```python
from build123d import *

# Parameters (mm, degrees)
SKETCH2_W           = 50.8
SKETCH2_H           = 25.4
BOSS_EXTRUDE1_DEPTH = 3.175
SKETCH4_W           = 38.1
SKETCH4_H           = 50.8
BOSS_EXTRUDE2_DEPTH = 3.175
SKETCH5_R           = 1.1
CUT_EXTRUDE1_DEPTH  = 3.175
SKETCH6_R           = 3.175
CUT_EXTRUDE2_DEPTH  = 3.175
BOSS_EXTRUDE3_DEPTH = 1.5875
FILLET3_R           = 1.5


with BuildPart() as part:
    # Sketch2 → Boss-Extrude1 (new body)
    with BuildSketch(Plane(origin=(0, 0, 0), x_dir=(0, 0, -1), z_dir=(1, 0, 0))):
        Rectangle(SKETCH2_W, SKETCH2_H)
    extrude(amount=BOSS_EXTRUDE1_DEPTH)

    # Sketch4 → Boss-Extrude2 (add)
    with BuildSketch(Plane(origin=(0, 12.7, 0), x_dir=(1, 0, 0), z_dir=(0, 1, 0))):
        with Locations((19.05, 0)):
            Rectangle(SKETCH4_W, SKETCH4_H)
    extrude(amount=-BOSS_EXTRUDE2_DEPTH)

    # Sketch5 → Cut-Extrude1 (cut)
    with BuildSketch(Plane(origin=(0, 12.7, 0), x_dir=(1, 0, 0), z_dir=(0, 1, 0))):
        with Locations(Location((8.05, 18.5, 0), (0, 0, 270))):
            Circle(SKETCH5_R)
        with Locations(Location((34.05, 18.5, 0), (0, 0, 270))):
            Circle(SKETCH5_R)
        with Locations(Location((34.05, -18.5, 0), (0, 0, 270))):
            Circle(SKETCH5_R)
        with Locations(Location((8.05, -18.5, 0), (0, 0, 270))):
            Circle(SKETCH5_R)
    extrude(amount=-CUT_EXTRUDE1_DEPTH, mode=Mode.SUBTRACT)

    # Sketch6 → Cut-Extrude2 (cut)
    with BuildSketch(Plane.ZY):
        with Locations((-12.7, 0)):
            Circle(SKETCH6_R)
        with Locations((12.7, 0)):
            Circle(SKETCH6_R)
    extrude(amount=-CUT_EXTRUDE2_DEPTH, mode=Mode.SUBTRACT)

    # Sketch7 → Boss-Extrude3 (add, symmetric)
    with BuildSketch(Plane.XY):
        Polygon((3.175, -12.7), (25.4, 9.525), (3.175, 9.525), align=None)
    extrude(amount=BOSS_EXTRUDE3_DEPTH, both=True)

    # Fillet3
    # the kernel refuses this fillet: 1.5 mm, written as the material it adds along each edge
    with BuildSketch(Plane(origin=(4.675, 8.025, 3.0875), x_dir=(-1, 0, 0), z_dir=(0, 1, 0))) as fillet3_piece_1_section:
        Polygon((0, 0), (FILLET3_R, 0), (FILLET3_R, -FILLET3_R), (0, -FILLET3_R), align=None)
    fillet3_piece_1 = extrude(amount=FILLET3_R, mode=Mode.PRIVATE)
    fillet3_piece_1 = fillet3_piece_1 - Plane(origin=(4.675, 8.025, 3.0875), x_dir=(0.7071067811865475, 0, 0.7071067811865475), z_dir=(0, 1, 0)) * Sphere(FILLET3_R, mode=Mode.PRIVATE)
    add(fillet3_piece_1)
    with BuildSketch(Plane(origin=(4.675, 8.025, -3.0875), x_dir=(0, 0, 1), z_dir=(0, 1, 0))) as fillet3_piece_2_section:
        Polygon((0, 0), (FILLET3_R, 0), (FILLET3_R, -FILLET3_R), (0, -FILLET3_R), align=None)
    fillet3_piece_2 = extrude(amount=FILLET3_R, mode=Mode.PRIVATE)
    fillet3_piece_2 = fillet3_piece_2 - Plane(origin=(4.675, 8.025, -3.0875), x_dir=(0.7071067811865475, 0, -0.7071067811865475), z_dir=(0, 1, 0)) * Sphere(FILLET3_R, mode=Mode.PRIVATE)
    add(fillet3_piece_2)
    with BuildSketch(Plane(origin=(3.175, 9.525, 25.4), x_dir=(0, -1, 0), z_dir=(0, 0, -1)), Plane(origin=(3.175, 9.525, -3.0875), x_dir=(0, -1, 0), z_dir=(0, 0, -1))) as fillet3_piece_3:
        with BuildLine():
            CenterArc((FILLET3_R, -FILLET3_R), FILLET3_R, 90, 90)
            Line((0, -FILLET3_R), (0, 0))
            Line((0, 0), (FILLET3_R, 0))
        make_face()
    extrude(amount=22.3125)
    with BuildSketch(Plane(origin=(29.15, 9.525, -1.5875), x_dir=(0, 0, -1), z_dir=(-1, 0, 0))) as fillet3_piece_4_section:
        with BuildLine():
            CenterArc((FILLET3_R, FILLET3_R), FILLET3_R, 180, 90)
            Line((0, FILLET3_R), (0, 0))
            Line((0, 0), (FILLET3_R, 0))
        make_face()
    fillet3_piece_4 = extrude(amount=24.475, mode=Mode.PRIVATE)
    fillet3_piece_4 = split(fillet3_piece_4, bisect_by=Plane(origin=(19.967902823, 4.092902823, -1.930123153), z_dir=(-0.707106781186549, 0.707106781186546, 0)), keep=Keep.TOP, mode=Mode.PRIVATE)
    add(fillet3_piece_4)
    with BuildSketch(Plane(origin=(25.4, 9.525, -1.5875), x_dir=(-0.7071067811865489, -0.7071067811865461, 0), z_dir=(0, 0, 1))) as fillet3_piece_5:
        with BuildLine():
            CenterArc((FILLET3_R * 0.414213562373, FILLET3_R), FILLET3_R, 225, 45)
            Line((-FILLET3_R * 0.292893218813, FILLET3_R * 0.292893218813), (0, 0))
            Line((0, 0), (FILLET3_R * 0.414213562373, 0))
        make_face()
    extrude(amount=3.175)
    with BuildSketch(Plane(origin=(3.175, 8.025, -1.5875), x_dir=(0, 0, -1), z_dir=(0, -1, 0))) as fillet3_piece_6_section:
        with BuildLine():
            CenterArc((FILLET3_R, FILLET3_R), FILLET3_R, 180, 90)
            Line((0, FILLET3_R), (0, 0))
            Line((0, 0), (FILLET3_R, 0))
        make_face()
    fillet3_piece_6 = extrude(amount=20.725, mode=Mode.PRIVATE)
    fillet3_piece_6 = split(fillet3_piece_6, bisect_by=Plane(origin=(8.60741784, -7.26758216, -1.930100054), z_dir=(-0.707106781186549, 0.707106781186546, 0)), keep=Keep.TOP, mode=Mode.PRIVATE)
    add(fillet3_piece_6)
    with BuildSketch(Plane(origin=(29.15, 9.525, 1.5875), x_dir=(0, 0, 1), z_dir=(-1, 0, 0))) as fillet3_piece_7_section:
        with BuildLine():
            CenterArc((FILLET3_R, -FILLET3_R), FILLET3_R, 90, 90)
            Line((0, -FILLET3_R), (0, 0))
            Line((0, 0), (FILLET3_R, 0))
        make_face()
    fillet3_piece_7 = extrude(amount=24.475, mode=Mode.PRIVATE)
    fillet3_piece_7 = split(fillet3_piece_7, bisect_by=Plane(origin=(19.967902823, 4.092902823, 1.930123153), z_dir=(-0.707106781186549, 0.707106781186546, 0)), keep=Keep.TOP, mode=Mode.PRIVATE)
    add(fillet3_piece_7)
    with BuildSketch(Plane(origin=(3.175, 8.025, 1.5875), x_dir=(0, 0, 1), z_dir=(0, -1, 0))) as fillet3_piece_8_section:
        with BuildLine():
            CenterArc((FILLET3_R, -FILLET3_R), FILLET3_R, 90, 90)
            Line((0, -FILLET3_R), (0, 0))
            Line((0, 0), (FILLET3_R, 0))
        make_face()
    fillet3_piece_8 = extrude(amount=20.725, mode=Mode.PRIVATE)
    fillet3_piece_8 = split(fillet3_piece_8, bisect_by=Plane(origin=(8.60741784, -7.26758216, 1.930100054), z_dir=(-0.707106781186549, 0.707106781186546, 0)), keep=Keep.TOP, mode=Mode.PRIVATE)
    add(fillet3_piece_8)
    with BuildSketch(Plane(origin=(25.4, 9.525, -3.140800859), x_dir=(-0.7071067811865446, -0.7071067811865503, 0), z_dir=(0, 0, 1))) as fillet3_piece_9a_section:
        with BuildLine():
            CenterArc((FILLET3_R * 0.414213562373, FILLET3_R), FILLET3_R, 225, 45)
            Line((-FILLET3_R * 0.292893218813, FILLET3_R * 0.292893218813), (0, 0))
            Line((0, 0), (FILLET3_R * 0.414213562373, 0))
        make_face()
    fillet3_piece_9a = extrude(amount=4.728300859, mode=Mode.PRIVATE)
    fillet3_piece_9a = split(fillet3_piece_9a, bisect_by=Plane(origin=(25.438403899, 9.432284787, -1.5875), z_dir=(0, 0, -1)), keep=Keep.TOP, mode=Mode.PRIVATE)
    with BuildSketch(Plane(origin=(29.15, 9.525, -1.5875), x_dir=(0, 0, -1), z_dir=(-1, 0, 0))) as fillet3_piece_9b_section:
        with BuildLine():
            CenterArc((FILLET3_R, FILLET3_R), FILLET3_R, 180, 90)
            Line((0, FILLET3_R), (0, 0))
            Line((0, 0), (FILLET3_R, 0))
        make_face()
    fillet3_piece_9b = extrude(amount=24.475, mode=Mode.PRIVATE)
    fillet3_piece_9b = split(fillet3_piece_9b, bisect_by=Plane(origin=(26.063627713, 10.188627713, -1.91198662), z_dir=(0.707106781186549, -0.707106781186546, 0)), keep=Keep.TOP, mode=Mode.PRIVATE)
    fillet3_piece_9 = fillet3_piece_9a & fillet3_piece_9b
    add(fillet3_piece_9)
    with BuildSketch(Plane(origin=(25.4, 9.525, -1.5875), x_dir=(-0.7071067811865489, -0.7071067811865461, 0), z_dir=(0, 0, 1))) as fillet3_piece_10a_section:
        with BuildLine():
            CenterArc((FILLET3_R * 0.414213562373, FILLET3_R), FILLET3_R, 225, 45)
            Line((-FILLET3_R * 0.292893218813, FILLET3_R * 0.292893218813), (0, 0))
            Line((0, 0), (FILLET3_R * 0.414213562373, 0))
        make_face()
    fillet3_piece_10a = extrude(amount=4.728300859, mode=Mode.PRIVATE)
    fillet3_piece_10a = split(fillet3_piece_10a, bisect_by=Plane(origin=(25.438403899, 9.432284787, 1.5875), z_dir=(0, 0, 1)), keep=Keep.TOP, mode=Mode.PRIVATE)
    with BuildSketch(Plane(origin=(29.15, 9.525, 1.5875), x_dir=(0, 0, 1), z_dir=(-1, 0, 0))) as fillet3_piece_10b_section:
        with BuildLine():
            CenterArc((FILLET3_R, -FILLET3_R), FILLET3_R, 90, 90)
            Line((0, -FILLET3_R), (0, 0))
            Line((0, 0), (FILLET3_R, 0))
        make_face()
    fillet3_piece_10b = extrude(amount=24.475, mode=Mode.PRIVATE)
    fillet3_piece_10b = split(fillet3_piece_10b, bisect_by=Plane(origin=(26.063627713, 10.188627713, 1.91198662), z_dir=(0.707106781186549, -0.707106781186546, 0)), keep=Keep.TOP, mode=Mode.PRIVATE)
    fillet3_piece_10 = fillet3_piece_10a & fillet3_piece_10b
    add(fillet3_piece_10)
    # the kernel refuses this fillet: 1.5 mm, written as the material it takes off along each edge
    with BuildSketch(Plane(origin=(38.1, 16.45, 25.4), x_dir=(0, 0, -1), z_dir=(0, -1, 0)), Plane(origin=(-3.75, -12.7, -25.4), x_dir=(0, 0, 1), z_dir=(1, 0, 0))) as fillet3_2_piece_1:
        with BuildLine():
            CenterArc((FILLET3_R, -FILLET3_R), FILLET3_R, 90, 90)
            Line((0, -FILLET3_R), (0, 0))
            Line((0, 0), (FILLET3_R, 0))
        make_face()
    extrude(amount=10.675, mode=Mode.SUBTRACT)
    with BuildSketch(Plane(origin=(38.1, 16.45, -25.4), x_dir=(0, 0, 1), z_dir=(0, -1, 0)), Plane(origin=(-3.75, -12.7, 25.4), x_dir=(0, 0, -1), z_dir=(1, 0, 0))) as fillet3_2_piece_2:
        with BuildLine():
            CenterArc((FILLET3_R, FILLET3_R), FILLET3_R, 180, 90)
            Line((0, FILLET3_R), (0, 0))
            Line((0, 0), (FILLET3_R, 0))
        make_face()
    extrude(amount=10.675, mode=Mode.SUBTRACT)


solid = part.part
```
The listing builds one solid part. Answer for the finished solid, in the listing's coordinates (mm). A direction names the side the tool comes from. Round coordinates to 2 decimals unless told otherwise and drop trailing zeros. Loops run counter-clockwise (first coordinate to the right, second up) from the corner with the lowest first, then second, coordinate; pieces in that order, holes last.
1) A cutting plane is placed at D-D on x = 34.05. Determine the outline of the cut face in (y, z) (3 decimals).
Outcome:
outline: (9.525, -25.4) - (12.7, -25.4) - (12.7, -19.6) - (9.525, -19.6) - close; (9.525, -17.4) - (12.7, -17.4) - (12.7, 17.4) - (9.525, 17.4) - close; (9.525, 19.6) - (12.7, 19.6) - (12.7, 25.4) - (9.525, 25.4) - close
2) Given P1, Ø6, axis at y = 1, z = -11, coming from the +X side (3 decimals); P2, Ø3, axis at x = 8.05, z = -18.5, coming from the -Y side (3 decimals); P3, Ø10, axis at y = 3, z = 7.5, coming from the +X side; P4, Ø4, axis at y = 0, z = 12.7, coming from the -X side, each flat-ended and moving along its own axis, determine where each tip first touches the part or whether it passes through.
Outcome:
P1: stops at x = 3.175
P2: stops at y = 9.525
P3: stops at x = 3.29
P4: passes through
3) Consider line 1 (X direction, y = 10.85, z = 18.5); line 2 (X direction, y = 11.5, z = 19); line 3 (Y direction, x = 2.05, z = 12.7) (3 decimals). Determine where each line is inside the solid, lowest interval first.
Outcome:
line 1: x = 0 to 6.95, 9.15 to 32.95, 35.15 to 38.1
line 2: x = 0 to 7.07, 9.03 to 33.07, 35.03 to 38.1
line 3: y = -12.7 to -3.175, 3.175 to 12.7
4) For a pull along X with two mould halves and no side action, classify faces 1 (the face through (10, 2, 1.588)), 2 (the face through (8.1, 11.1, -19.6)), 3 (the face through (8.1, 11.1, 17.4)), 4 (the face through (25.45, 9.41, -0.04)) as released by +X, released by -X, zero draft, split by the parting line, or undercut.
Outcome:
face 1: zero draft
face 2: undercut
face 3: undercut
face 4: released by +X
5) A cutting plane is placed at A-A on z = 12.7. Determine the outline of the cut face in (x, y) (3 decimals), plus the area to 3 significant figures.
Outcome:
outline: (0, -12.7) - (3.175, -12.7) - (3.175, -3.175) - (0, -3.175) - close; (0, 3.175) - (3.175, 3.175) - (3.175, 8.025) arc R1.5 cw to (4.675, 9.525) - (38.1, 9.525) - (38.1, 12.7) - (0, 12.7) - close
area: 172 mm2
6) For faces 5 (the face through (3.626, -2.192, -2.015)), 6 (the face through (21, 9.525, -6)), 7 (the face through (34.1, 11.1, 17.4)), 8 (the face through (3.175, -4, 14)), 9 (the face through (38.1, 11, 0)), determine the directions among +Z, -Z, +X, -X, +Y, -Y from which every point of the face is accessible in a straight line to the end or side of a thin tool.
Outcome:
face 5: -Z, +X, -Y
face 6: +X, -Y
face 7: +Y, -Y
face 8: +Z, +X, -Y
face 9: +Z, -Z, +X, +Y, -Y
7) A cutting plane is placed at B-B on y = 0. Determine the outline of the cut face in (x, z) (1 decimal), plus the area to 3 significant figures.
Outcome:
outline: (0, -25.4) - (3.2, -25.4) - (3.2, -15.9) - (0, -15.9) - close; (0, -9.5) - (3.2, -9.5) - (3.2, -3.1) arc R1.5 cw to (4.7, -1.6) - (15.9, -1.6) - (15.9, 1.6) - (4.7, 1.6) arc R1.5 cw to (3.2, 3.1) - (3.2, 9.5) - (0, 9.5) - close; (0, 15.9) - (3.2, 15.9) - (3.2, 25.4) - (0, 25.4) - close
area: 162 mm2
8) A cutting plane is placed at C-C on z = -18.5. Determine the outline of the cut face in (x, y) (3 decimals).
Outcome:
outline: (0, -12.7) - (3.175, -12.7) - (3.175, 8.025) arc R1.5 cw to (4.675, 9.525) - (6.95, 9.525) - (6.95, 12.7) - (0, 12.7) - close; (9.15, 9.525) - (32.95, 9.525) - (32.95, 12.7) - (9.15, 12.7) - close; (35.15, 9.525) - (38.1, 9.525) - (38.1, 12.7) - (35.15, 12.7) - close
